```python
from build123d import *

# Parameters (mm, degrees)
F_3_8_CLEARANCE_HOLE1_D                = 10.0838
CIRPATTERN1_COUNT                      = 10
SKETCH5_RX                             = 50.8
SKETCH5_RY                             = 31.75
CUT_EXTRUDE1_DEPTH                     = 2.032
SKETCH6_R                              = 0.635
CUT_EXTRUDE2_DEPTH                     = 108.849548557
F_1_8_0_125_DIAMETER_HOLE1_D           = 3.175
F_1_8_0_125_DIAMETER_HOLE1_DEPTH       = 2.856133767
F_1_8_0_125_DIAMETER_HOLE1_CSINK_D     = 3.81
F_1_8_0_125_DIAMETER_HOLE1_CSINK_ANGLE = 90
F_1_8_0_125_DIAMETER_HOLE1_TIP         = 0.953866233


with BuildPart() as part:
    # Sketch1 → Revolve1 (revolve)
    with BuildSketch(Plane.XY, mode=Mode.PRIVATE) as revolve1_sk:
        Polygon((0, -6.35), (54.8259, -6.35), (54.8259, -3.6576), (58.8899, -3.6576), (58.8899, -6.35), (76.2, -6.35), (76.2, 0), (0, 0), align=None)
    revolve(revolve1_sk.sketch.rotate(Axis((0, 0, 0), (0, -1, 0)), 90), axis=Axis((0, 0, 0), (0, -1, 0)))

    # 3/8 Clearance Hole1 (through all)
    with Locations(Plane(origin=(67.31, 0, 0), x_dir=(0, 0, 1), z_dir=(0, 1, 0))):
        with Locations((0, 0)):
            f_3_8_clearance_hole1 = Hole(F_3_8_CLEARANCE_HOLE1_D / 2)

    # CirPattern1: 3/8 Clearance Hole1 ×10 about axis
    cirpattern1_axis = Axis((0, 0, 0), (0, 1, 0))
    for i in range(1, CIRPATTERN1_COUNT):
        add(f_3_8_clearance_hole1.rotate(cirpattern1_axis, i * 360 / CIRPATTERN1_COUNT), mode=Mode.SUBTRACT)

    # Sketch5 → Cut-Extrude1 (cut)
    with BuildSketch(Plane(origin=(0, 0, 0), x_dir=(1, 0, 0), z_dir=(0, 1, 0))):
        with Locations((0, 0)):
            Ellipse(SKETCH5_RX, SKETCH5_RY)
        with BuildLine():
            Line((-3.302199606, -2.201466404), (-28.702199606, 35.898533596))
            ThreePointArc((-28.702199606, 35.898533596), (-27.601466404, 41.402199606), (-22.097800394, 40.301466404))
            Line((-22.097800394, 40.301466404), (3.302199606, 2.201466404))
            ThreePointArc((3.302199606, 2.201466404), (2.201466404, -3.302199606), (-3.302199606, -2.201466404))
        make_face()
    extrude(amount=-CUT_EXTRUDE1_DEPTH, mode=Mode.SUBTRACT)

    # Sketch6 → Cut-Extrude2 (cut, through all)
    with BuildSketch(Plane(origin=(0, -2.032, 0), x_dir=(1, 0, 0), z_dir=(0, 1, 0))):
        with Locations(Location((-5.1816, -8.974794464, 0), (0, 0, 270))):
            Circle(SKETCH6_R)
        with Locations(Location((5.1816, -8.974794464, 0), (0, 0, 270))):
            Circle(SKETCH6_R)
        with Locations(Location((24.511, 0, 0), (0, 0, 270))):
            Circle(SKETCH6_R)
        with Locations(Location((18.2118, 0, 0), (0, 0, 270))):
            Circle(SKETCH6_R)
        with Locations(Location((10.3632, 0, 0), (0, 0, 270))):
            Circle(SKETCH6_R)
        with Locations(Location((0, -18.2118, 0), (0, 0, 270))):
            Circle(SKETCH6_R)
        with Locations(Location((9.1059, -15.771881449, 0), (0, 0, 270))):
            Circle(SKETCH6_R)
        with Locations(Location((15.771881449, -9.1059, 0), (0, 0, 270))):
            Circle(SKETCH6_R)
        with Locations(Location((5.1816, 8.974794464, 0), (0, 0, 270))):
            Circle(SKETCH6_R)
        with Locations(Location((-5.1816, 8.974794464, 0), (0, 0, 270))):
            Circle(SKETCH6_R)
        with Locations(Location((-10.3632, 0, 0), (0, 0, 270))):
            Circle(SKETCH6_R)
        with Locations(Location((15.771881449, 9.1059, 0), (0, 0, 270))):
            Circle(SKETCH6_R)
        with Locations(Location((9.1059, 15.771881449, 0), (0, 0, 270))):
            Circle(SKETCH6_R)
        with Locations(Location((0, 18.2118, 0), (0, 0, 270))):
            Circle(SKETCH6_R)
        with Locations(Location((-9.1059, 15.771881449, 0), (0, 0, 270))):
            Circle(SKETCH6_R)
        with Locations(Location((-15.771881449, 9.1059, 0), (0, 0, 270))):
            Circle(SKETCH6_R)
        with Locations(Location((-18.2118, 0, 0), (0, 0, 270))):
            Circle(SKETCH6_R)
        with Locations(Location((-15.771881449, -9.1059, 0), (0, 0, 270))):
            Circle(SKETCH6_R)
        with Locations(Location((-9.1059, -15.771881449, 0), (0, 0, 270))):
            Circle(SKETCH6_R)
        with Locations(Location((-6.343913615, -23.675807928, 0), (0, 0, 270))):
            Circle(SKETCH6_R)
        with Locations(Location((0, -24.511, 0), (0, 0, 270))):
            Circle(SKETCH6_R)
        with Locations(Location((6.343913615, -23.675807928, 0), (0, 0, 270))):
            Circle(SKETCH6_R)
        with Locations(Location((12.2555, -21.227148672, 0), (0, 0, 270))):
            Circle(SKETCH6_R)
        with Locations(Location((17.331894314, -17.331894314, 0), (0, 0, 270))):
            Circle(SKETCH6_R)
        with Locations(Location((21.227148672, -12.2555, 0), (0, 0, 270))):
            Circle(SKETCH6_R)
        with Locations(Location((23.675807928, -6.343913615, 0), (0, 0, 270))):
            Circle(SKETCH6_R)
        with Locations(Location((-17.331894314, 17.331894314, 0), (0, 0, 270))):
            Circle(SKETCH6_R)
        with Locations(Location((-21.227148672, 12.2555, 0), (0, 0, 270))):
            Circle(SKETCH6_R)
        with Locations(Location((-23.675807928, 6.343913615, 0), (0, 0, 270))):
            Circle(SKETCH6_R)
        with Locations(Location((-24.511, 0, 0), (0, 0, 270))):
            Circle(SKETCH6_R)
        with Locations(Location((-23.675807928, -6.343913615, 0), (0, 0, 270))):
            Circle(SKETCH6_R)
        with Locations(Location((-21.227148672, -12.2555, 0), (0, 0, 270))):
            Circle(SKETCH6_R)
        with Locations(Location((-17.331894314, -17.331894314, 0), (0, 0, 270))):
            Circle(SKETCH6_R)
        with Locations(Location((-12.2555, -21.227148672, 0), (0, 0, 270))):
            Circle(SKETCH6_R)
        with Locations(Location((23.675807928, 6.343913615, 0), (0, 0, 270))):
            Circle(SKETCH6_R)
        with Locations(Location((21.227148672, 12.2555, 0), (0, 0, 270))):
            Circle(SKETCH6_R)
        with Locations(Location((17.331894314, 17.331894314, 0), (0, 0, 270))):
            Circle(SKETCH6_R)
        with Locations(Location((12.2555, 21.227148672, 0), (0, 0, 270))):
            Circle(SKETCH6_R)
        with Locations(Location((6.343913615, 23.675807928, 0), (0, 0, 270))):
            Circle(SKETCH6_R)
        with Locations(Location((0, 24.511, 0), (0, 0, 270))):
            Circle(SKETCH6_R)
        with Locations(Location((-6.343913615, 23.675807928, 0), (0, 0, 270))):
            Circle(SKETCH6_R)
        with Locations(Location((-12.2555, 21.227148672, 0), (0, 0, 270))):
            Circle(SKETCH6_R)
    extrude(amount=-CUT_EXTRUDE2_DEPTH, mode=Mode.SUBTRACT)

    # 1/8 (0.125) Diameter Hole1
    with Locations(Plane(origin=(0, 0, -45.72), x_dir=(0, 0, 1), z_dir=(0, 1, 0))):
        with Locations((0, 0), (91.44, 0)):
            CounterSinkHole(F_1_8_0_125_DIAMETER_HOLE1_D / 2, F_1_8_0_125_DIAMETER_HOLE1_CSINK_D / 2, depth=F_1_8_0_125_DIAMETER_HOLE1_DEPTH, counter_sink_angle=F_1_8_0_125_DIAMETER_HOLE1_CSINK_ANGLE)
            with Locations((0, 0, -(F_1_8_0_125_DIAMETER_HOLE1_DEPTH + F_1_8_0_125_DIAMETER_HOLE1_TIP / 2))):  # 118° drill point
                Cone(0, F_1_8_0_125_DIAMETER_HOLE1_D / 2, F_1_8_0_125_DIAMETER_HOLE1_TIP, mode=Mode.SUBTRACT)


solid = part.part
```
Can you work these out from the model? Positions are in its coordinate system, mm. A direction names the side the tool comes from. Give positions to 0.01 mm unless a question says otherwise; leave off trailing zeros. Write each loop counter-clockwise with the first axis right and the second up, starting at its lowest first coordinate (ties: lowest second). Pieces come first, ordered by that corner, then holes. Notation, with made-up numbers: (-7, 79) - (49, 79) arc R19 ccw to (49, 86) - close; hole circle Ø4 at (30.25, 22). An arc over 180 degrees is marked (long way). Write item = value, one per line. Start each with the question number.
1. Imagine slicing it at A-A (x = 67.31). Please give me the cut outline in (y, z), and give its area (3 significant figures).
2. On a 3-axis mill with a long thin cutter (end or side, diameter ignored), from which of +Z, -Z, +X, -X, +Y, -Y can I reach the whole of each face in a straight line? I mean faces 4 (the face through (-18.796, -1.002, -35.349)), 5 (the face through (-1, 0, 33)), 6 (the face through (33.36, -4.98, -43.51)). Say none if no direction works.
3. Imagine slicing it at B-B (z = -38.1). Please give me the cut outline in (x, y), and give its area (3 significant figures).
4. For pin 1 (1.5 mm diameter, centred on x = 10.36, z = 0, fed in from +Y); pin 2 (3 mm diameter, centred on x = -48.5, y = -5.5, fed in from -Z); pin 3 (2 mm diameter, centred on y = -5, z = 51, fed in from -X), each with a flat end and sliding along its axis, tell me the tip position at first contact or that it passes through.
5. Please list where these lines run through material, in increasing order: line 1 (Z direction, x = 53, y = -2.5); line 2 (X direction, y = -4, z = -10); line 3 (X direction, y = -4, z = 34).
6. Thinking about a two-plate mould opening in Z: for faces 1 (the face through (-26.079, -1.002, -31.964)), 2 (the face through (74.388, -3.131, -16.519)), 3 (the face through (-1, -6.35, 1)), which applies, released by +Z, released by -Z, zero draft, split by the parting line, or undercut?
Worked answers:
q1.outline = (-6.35, -35.72) - (0, -35.72) - (0, -5.04) - (-6.35, -5.04) - close; (-6.35, 5.04) - (0, 5.04) - (0, 35.72) - (-6.35, 35.72) - close
q1.area = 390 mm2
q2.face_4 = +Y
q2.face_5 = +Z, -Z, +X, -X, +Y
q2.face_6 = -Y
q3.outline = (-65.99, -6.35) - (-59.28, -6.35) - (-59.28, 0) - (-65.99, 0) - close; (-49.63, -6.35) - (-44.9, -6.35) - (-44.9, -3.66) - (-39.42, -3.66) - (-39.42, -6.35) - (39.42, -6.35) - (39.42, -3.66) - (44.9, -3.66) - (44.9, -6.35) - (49.63, -6.35) - (49.63, 0) - (-20.63, 0) - (-20.63, -2.03) - (-29.37, -2.03) - (-29.37, 0) - (-49.63, 0) - close; (59.28, -6.35) - (65.99, -6.35) - (65.99, 0) - (59.28, 0) - close
q3.area = 668 mm2
q4.pin_1 = -2.03
q4.pin_2 = -59.98
q4.pin_3 = -57.5
q5.line_1 = -54.75 to -44.39, -34.74 to 34.74, 44.39 to 54.75
q5.line_2 = -75.54 to -58.03, -53.91 to 53.91, 58.03 to 75.54
q5.line_3 = -68.19 to -48.08, -43.01 to 43.01, 48.08 to 68.19
q6.face_1 = undercut
q6.face_2 = split by the parting line
q6.face_3 = zero draft
